Input: part model. Units: mm. Frame: model coordinates. A direction names the side the tool comes from. Give positions to 0.01 mm unless a question says otherwise; leave off trailing zeros. Order: outer loops, then holes, each group sorted by start corner. A loop starts at its lowest first (then second) coordinate and runs counter-clockwise, first axis right, second up.
Autodesk Inventor part; units mm, degrees
ref_plane "YZ Plane" through (0, 0, 0) normal (1, 0, 0) x (0, 1, 0)
ref_plane "XZ Plane" through (0, 0, 0) normal (0, 1, 0) x (-1, 0, 0)
ref_plane "XY Plane" through (0, 0, 0) normal (0, 0, 1) x (1, 0, 0)
sketch "Sketch1" plane through (0, 0, 0) normal (0, 1, 0) x (-1, 0, 0)
  line L0 (-18.95, -18.95) -> (18.95, -18.95)
  line L1 (18.95, -18.95) -> (18.95, 18.95)
  line L2 (18.95, 18.95) -> (-18.95, 18.95)
  line L3 (-18.95, 18.95) -> (-18.95, -18.95)
  line L4 (-18.95, -18.95) -> (18.95, 18.95) construction
  line L5 (18.95, -18.95) -> (-18.95, 18.95) construction
  line L6 (-2.45, -13.45) -> (2.45, -13.45) construction
  line L7 (2.45, -13.45) -> (2.45, 13.45) construction
  line L8 (2.45, 13.45) -> (-2.45, 13.45) construction
  line L9 (-2.45, 13.45) -> (-2.45, -13.45) construction
  line L10 (-2.45, -13.45) -> (2.45, 13.45) construction
  line L11 (2.45, -13.45) -> (-2.45, 13.45) construction
  line L12 (-13.45, -2.45) -> (13.45, -2.45) construction
  line L13 (13.45, -2.45) -> (13.45, 2.45) construction
  line L14 (13.45, 2.45) -> (-13.45, 2.45) construction
  line L15 (-13.45, 2.45) -> (-13.45, -2.45) construction
  line L16 (-13.45, -2.45) -> (13.45, 2.45) construction
  line L17 (13.45, -2.45) -> (-13.45, 2.45) construction
  line L18 (-13.6, -2.6) -> (13.6, -2.6)
  line L19 (13.6, -2.6) -> (13.6, 2.6)
  line L20 (13.6, 2.6) -> (-13.6, 2.6)
  line L21 (-13.6, 2.6) -> (-13.6, -2.6)
  line L22 (-13.6, -2.6) -> (13.6, 2.6) construction
  line L23 (13.6, -2.6) -> (-13.6, 2.6) construction
  line L24 (-2.6, -13.6) -> (2.6, -13.6)
  line L25 (2.6, -13.6) -> (2.6, 13.6)
  line L26 (2.6, 13.6) -> (-2.6, 13.6)
  line L27 (-2.6, 13.6) -> (-2.6, -13.6)
  line L28 (-2.6, -13.6) -> (2.6, 13.6) construction
  line L29 (2.6, -13.6) -> (-2.6, 13.6) construction
  point P0 (0, 0)
  point P1 (0, 0)
  dimension "d0" = 37.9
  dimension "d1" = 4.9
  dimension "d2" = 11
  dimension "d3" = 0.15
  dimension "d4" = 0.15
extrude "Extrusion1" add sketch "Sketch1" along normal blind 1.9
sketch "Sketch2" plane through (0, 1.9, 0) normal (0, 1, 0) x (1, 0, 0)
  line L0 (18.95, 18.95) -> (-18.95, 18.95)
  line L1 (-18.95, 18.95) -> (-18.95, -18.95)
  line L2 (-18.95, -18.95) -> (18.95, -18.95)
  line L3 (18.95, -18.95) -> (18.95, 18.95)
  circle A0 centre (0, 0) radius 1.5
  dimension "d7" = 3
extrude "Extrusion2" add sketch "Sketch2" along normal blind 2
sketch "Sketch3" plane through (0, 3.9, 0) normal (0, 1, 0) x (1, 0, 0)
  circle A0 centre (0, 0) radius 1.5
  line L0 (18.95, 18.95) -> (-18.95, 18.95)
  line L1 (-18.95, 18.95) -> (-18.95, -18.95)
  line L2 (-18.95, -18.95) -> (18.95, -18.95)
  line L3 (18.95, -18.95) -> (18.95, 18.95)
  circle A1 centre (0, 0) radius 2.75
  dimension "d10" = 5.5
extrude "Extrusion3" add sketch "Sketch3" along normal blind 2.5 contours L3 L2 L1 L0
chamfer "Chamfer1" distance 2 angle 45 1 edges at (-2.6, 0.95, -2.6)
fillet "Fillet1" radius 2.45 1 edges at (-13.6, 0.95, -2.6)
fillet "Fillet2" radius 2.45 1 edges at (-2.6, 0.95, -13.6)
chamfer "Chamfer2" distance 2 angle 45 1 edges at (2.6, 0.95, -2.6)
chamfer "Chamfer3" distance 2 angle 45 1 edges at (2.6, 0.95, 2.6)
fillet "Fillet3" radius 2.45 1 edges at (13.6, 0.95, -2.6)
fillet "Fillet4" radius 2.45 1 edges at (2.6, 0.95, -13.6)
fillet "Fillet5" radius 2.45 1 edges at (13.6, 0.95, 2.6)
fillet "Fillet6" radius 2.45 1 edges at (2.6, 0.95, 13.6)
chamfer "Chamfer4" distance 2 angle 45 1 edges at (-2.6, 0.95, 2.6)
fillet "Fillet7" radius 2.45 2 edges at (-2.6, 0.95, 13.6) (-13.6, 0.95, 2.6)
equation "\"d0\" = 3 * ServoArmLength + ServoArmWidth"
equation "\"d1\" = ServoArmWidth"
equation "\"d2\" = ServoArmLength"
equation "\"d3\" = ServoArmSpacing"
equation "\"d4\" = ServoArmSpacing"
equation "\"d5\" = ServoArmThickness"
equation "\"d7\" = ServoArmHoleRequired"
equation "\"d8\" = MinimalThickness"
equation "\"d10\" = ServoArmHeadScrewTrace"
equation "\"d11\" = ServoArmHeadScrewThickness"
equation "\"d13\" = ServoArmInternFillet"
equation "\"d16\" = ServoArmExternFillet"
equation "\"d17\" = ServoArmExternFillet"
equation "\"d18\" = ServoArmInternFillet"
equation "\"d21\" = ServoArmInternFillet"
equation "\"d24\" = ServoArmExternFillet"
equation "\"d25\" = ServoArmExternFillet"
equation "\"d26\" = ServoArmExternFillet"
equation "\"d27\" = ServoArmExternFillet"
equation "\"d28\" = ServoArmInternFillet"
equation "\"d31\" = ServoArmExternFillet"
properties part number "ServoArmTrace"
1) Cut plane C-C (z = 1). Return the cut outline in (x, y), then the cut area to 3 significant figures.
2) Pull-direction query (X, two-part tool) for faces 1 (the face through (-12.901, 0.963, 1.863)), 2 (the face through (0, 3, -18.95)), 3 (the face through (-18.95, 3, 0)); classes: pulls with the +X half, pulls with the -X half, needs draft (parallel to the pull), parting line crosses it, or undercut.
3) First-contact query: P1, Ø5, axis at x = 0, z = 0, coming from the +Y side. Flat tip, straight axial feed; report the tip coordinate or a pass-through.
4) Line query: probe 1 along X at (y, z) = (4.4, 0); probe 2 along X at (y, z) = (3.2, 0). Output: solid intervals per line, ascending.
5) Cut plane B-B (z = -9). Return the cut outline in (x, y), then the cut area to 3 significant figures.
6) Reachability of faces 4 (the face through (-0.596, 5.132, -2.685)), 5 (the face through (2.6, 1, -8)), 6 (the face through (4, 0, 4)) from +Z, -Z, +X, -X, +Y, -Y: full face, straight path, thin tool, end or side. Return the list, or none.
7) Cut plane A-A (x = 5.5). Return the cut outline in (y, z).
8) Cut plane D-D (x = -2). Return the cut outline in (y, z), then the cut area to 3 significant figures.
Geometry says:
1. outline: (-18.95, 0) - (-13.45, 0) - (-13.45, 1.9) - (-1.12, 1.9) - (-1.12, 3.9) - (-2.56, 3.9) - (-2.56, 6.4) - (-18.95, 6.4) - close; (1.12, 1.9) - (13.45, 1.9) - (13.45, 0) - (18.95, 0) - (18.95, 6.4) - (2.56, 6.4) - (2.56, 3.9) - (1.12, 3.9) - close
1. area: 174 mm2
2. face 1: undercut
2. face 2: needs draft
2. face 3: pulls with the -X half
3. P1: stops at y = 3.9
4. probe 1: x = -18.95 to -2.75, 2.75 to 18.95
4. probe 2: x = -18.95 to -1.5, 1.5 to 18.95
5. outline: (-18.95, 0) - (-2.6, 0) - (-2.6, 1.9) - (2.6, 1.9) - (2.6, 0) - (18.95, 0) - (18.95, 6.4) - (-18.95, 6.4) - close
5. area: 233 mm2
6. face 4: +Y
6. face 5: -Y
6. face 6: +Z, -Z, +X, -X, -Y
7. outline: (0, -18.95) - (6.4, -18.95) - (6.4, 18.95) - (0, 18.95) - (0, 2.6) - (1.9, 2.6) - (1.9, -2.6) - (0, -2.6) - close
8. outline: (0, -18.95) - (6.4, -18.95) - (6.4, -1.89) - (3.9, -1.89) - (3.9, 1.89) - (6.4, 1.89) - (6.4, 18.95) - (0, 18.95) - (0, 12.76) - (1.9, 12.76) - (1.9, -12.76) - (0, -12.76) - close
8. area: 185 mm2
